Geometry: see drawing. Coordinates: mm, zero at the bounding-box minimum. A direction names the side the tool comes from. Coordinates: 2 decimals unless noted, no trailing zeros. Order: outer loops, then holes, each group sorted by start corner. A loop starts at its lowest first (then second) coordinate and runs counter-clockwise, first axis right, second up. Notation, with made-up numbers: (42.5, -33.75) -> (71.5, -33.75) arc R23 cw to (71.5, -14.75) -> close; hole circle Ø7 at (-14.5, 77). An arc over 180 degrees is marked (long way). Write each question's results on one line, items separated by ' | '. Start each with the question number.
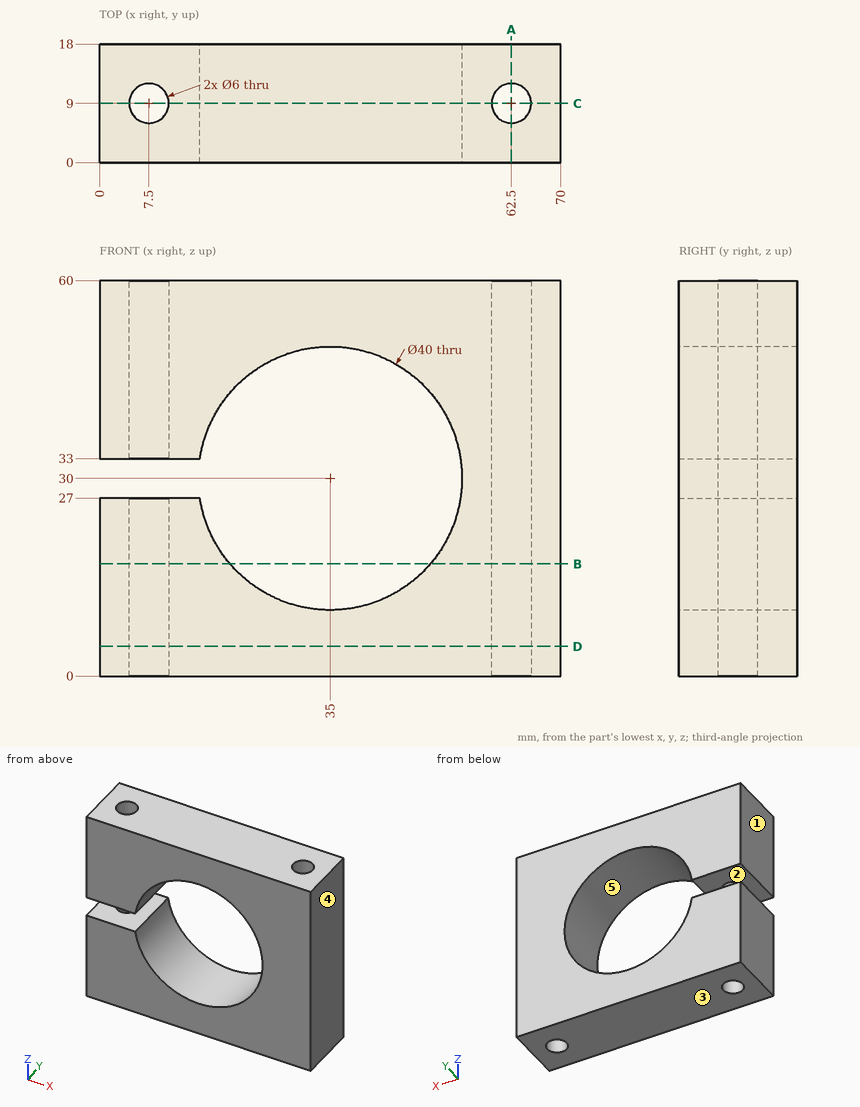
(1) Section C-C on y = 9. Return the cut outline in (x, z), then the cut area to 3 significant figures.
(2) Section D-D on z = 4.5. Return the cut outline in (x, y).
(3) Section B-B on z = 17. Return the cut outline in (x, y).
(4) Line query: L1, parallel to Y at x = 62.5, z = 17; L2, parallel to Z at x = 35, y = 5.25; L3, parallel to Z at x = 13.5, y = 15.75. Output: solid intervals per line, ascending.
(5) Section A-A on x = 62.5. Return the cut outline in (y, z), then the cut area to 3 significant figures.
(6) First-contact query: P1, Ø1, axis at x = 12, z = 44, coming from the -Y side; P2, Ø5, axis at x = 18.5, z = 32.5, coming from the -Y side. Flat tips, straight axial feed; report the tip coordinate or a pass-through.
(7) Draft query along Z for the marked faces 3, 4 and 5. Return one class per face: released by +Z, released by -Z, zero draft, split by the parting line, or undercut.
(8) Reachability of the marked faces 1 and 2 from +Z, -Z, +X, -X, +Y, -Y: full face, straight path, thin tool, end or side. Return the list, or none.
Results list:
1) outline: (0, 0) -> (4.5, 0) -> (4.5, 27) -> (0, 27) -> close; (0, 33) -> (4.5, 33) -> (4.5, 60) -> (0, 60) -> close; (10.5, 0) -> (59.5, 0) -> (59.5, 60) -> (10.5, 60) -> (10.5, 33) -> (15.23, 33) arc R20 cw (long way) to (15.23, 27) -> (10.5, 27) -> close; (65.5, 0) -> (70, 0) -> (70, 60) -> (65.5, 60) -> close | area: 2,170 mm²
2) outline: (0, 0) -> (70, 0) -> (70, 18) -> (0, 18) -> close; hole circle Ø6 at (7.5, 9); hole circle Ø6 at (62.5, 9)
3) outline: (0, 0) -> (19.8, 0) -> (19.8, 18) -> (0, 18) -> close; (50.2, 0) -> (70, 0) -> (70, 18) -> (50.2, 18) -> close; hole circle Ø6 at (7.5, 9); hole circle Ø6 at (62.5, 9)
4) L1: y = 0 to 6, 12 to 18 | L2: z = 0 to 10, 50 to 60 | L3: z = 0 to 27, 33 to 60
5) outline: (0, 0) -> (6, 0) -> (6, 60) -> (0, 60) -> close; (12, 0) -> (18, 0) -> (18, 60) -> (12, 60) -> close | area: 720 mm²
6) P1: stops at y = 0 | P2: passes through
7) face 3: released by -Z | face 4: zero draft | face 5: undercut
8) face 1: +Z, -Z, -X, +Y, -Y | face 2: -X, +Y, -Y
